from build123d import *

# Parameters (mm, degrees)
SKETCH_1_W          = 51.2
SKETCH_1_H          = 48
EXTRUDE_1_DEPTH     = 120
FILLET_1_R          = 10
SKETCH_3_R          = 6.803864169
EXTRUDE_2_DEPTH     = 10
SKETCH_4_R          = 32
EXTRUDE_3_DEPTH     = 32.5
SKETCH_5_W          = 48
SKETCH_5_H          = 35
CUT_EXTRUDE_1_DEPTH = 178.007598707
SKETCH_6_W          = 6
SKETCH_6_H          = 120
EXTRUDE_6_DEPTH     = 4


with BuildPart() as part:
    # Sketch 1 → Extrude 1 (new body)
    with BuildSketch(Plane(origin=(0, 0, 0), x_dir=(1, 0, 0), z_dir=(0, 1, 0))):
        with Locations((25.6, 24)):
            Rectangle(SKETCH_1_W, SKETCH_1_H)
    extrude(amount=EXTRUDE_1_DEPTH)

    # Fillet 1
    fillet_1_edges = [part.edges().sort_by_distance(p)[0] for p in [
        (51.2, 60, -48),
    ]]
    fillet(fillet_1_edges, radius=FILLET_1_R)

    # Sketch 3 → Extrude 2 (add)
    with BuildSketch(Plane.XZ):
        with Locations(Location((13, -12, 0), (0, 0, 270))):
            Circle(SKETCH_3_R)
    extrude_2 = extrude(amount=EXTRUDE_2_DEPTH)

    # Sketch 4 → Extrude 3 (add)
    with BuildSketch(Plane.XZ.offset(10)):
        with Locations(Location((13, -12, 0), (0, 0, 270))):
            Circle(SKETCH_4_R)
    extrude_3 = extrude(amount=EXTRUDE_3_DEPTH)

    # Mirror 1: Extrude 2, Extrude 3 across plane
    add(extrude_2.mirror(Plane(origin=(0, 60, 0), x_dir=(0, 0, 1), z_dir=(0, -1, 0))))
    add(extrude_3.mirror(Plane(origin=(0, 60, 0), x_dir=(0, 0, 1), z_dir=(0, -1, 0))))

    # Sketch 5 → Cut-Extrude 1 (cut, through all)
    with BuildSketch(Plane.ZY):
        with Locations((-24, 60)):
            Rectangle(SKETCH_5_W, SKETCH_5_H)
    extrude(amount=-CUT_EXTRUDE_1_DEPTH, mode=Mode.SUBTRACT)


with BuildPart() as cut_extrude_1_piece_1:
    # of the separate pieces the step leaves, piece 1, a body of its own (cut_extrude_1_pieces)
    add(part.part.solids().sort_by_distance((13, 130, -44))[0])



with BuildPart() as cut_extrude_1_piece_2:
    # of the separate pieces the step leaves, piece 2, a body of its own (cut_extrude_1_pieces)
    add(part.part.solids().sort_by_distance((51.2, 0, -38))[0])


with BuildPart() as cut_extrude_1_piece_1_1:
    add(cut_extrude_1_piece_1.part)

    add(cut_extrude_1_piece_2.part)  # Extrude 6 merges Cut-Extrude 1 piece 2
    # Sketch 6 → Extrude 6 (add)
    with BuildSketch(Plane.ZY):
        with Locations((-21, 60)):
            Rectangle(SKETCH_6_W, SKETCH_6_H)
    extrude(amount=EXTRUDE_6_DEPTH)


solid = cut_extrude_1_piece_1_1.part
Geometry check sheet. Reference: the model listing, model coordinates, mm. A direction names the side the tool comes from. Coordinates: 2 decimals unless noted, no trailing zeros. Write each loop counter-clockwise with the first axis right and the second up, starting at its lowest first coordinate (ties: lowest second). Pieces come first, ordered by that corner, then holes. Notation, with made-up numbers: (58, 89.25) -> (107, 89.25) arc R19 cw to (107, 108.25) -> close; hole circle Ø4 at (-10.75, -0.5). An arc over 180 degrees is marked (long way). One line per question, with ' | ' between items.
1. Set-up check for faces 1 (the flat face through (0, 98, -36)), 2 (the flat face through (25, 21, 0)), 3 (the flat face through (0, 60, -21)), 4 (the flat face through (-2, 59, -18)), 5 (the cylindrical face through (-15.39, -26.022, -26.766)): record each of +Z, -Z, +X, -X, +Y, -Y from which the full face is reachable in a straight line by a thin tool's end or side.
Answers:
face 1: -Z, -X | face 2: +Z, +X, -X | face 3: +Z, -Z, +X | face 4: +Z, -X | face 5: -Y
2. Cross-section at B-B on z = -12. Record the cut outline in (x, y), and give its area (3 significant figures).
Answers:
outline: (-19, -42.5) -> (45, -42.5) -> (45, -10) -> (19.8, -10) -> (19.8, 0) -> (51.2, 0) -> (51.2, 42.5) -> (0, 42.5) -> (0, 0) -> (6.2, 0) -> (6.2, -10) -> (-19, -10) -> close; (-19, 130) -> (6.2, 130) -> (6.2, 120) -> (0, 120) -> (0, 77.5) -> (51.2, 77.5) -> (51.2, 120) -> (19.8, 120) -> (19.8, 130) -> (45, 130) -> (45, 162.5) -> (-19, 162.5) -> close | area: 8,780 mm²
3. Cross-section at C-C on x = 3.5. Record the cut outline in (y, z).
Answers:
outline: (-42.5, -42.56) -> (-10, -42.56) -> (-10, 18.56) -> (-42.5, 18.56) -> close; (0, -48) -> (42.5, -48) -> (42.5, 0) -> (0, 0) -> close; (77.5, -48) -> (120, -48) -> (120, 0) -> (77.5, 0) -> close; (130, -42.56) -> (162.5, -42.56) -> (162.5, 18.56) -> (130, 18.56) -> close
4. Cross-section at D-D on y = 33.5. Record the cut outline in (x, z), and give its area (3 significant figures).
Answers:
outline: (-4, -24) -> (0, -24) -> (0, -48) -> (41.2, -48) arc R10 ccw to (51.2, -38) -> (51.2, 0) -> (0, 0) -> (0, -18) -> (-4, -18) -> close | area: 2,460 mm²
5. Thickness scan on probe 1 along Y at (x, z) = (15.5, -1); probe 2 along Y at (x, z) = (-13.5, -29.5); probe 3 along Y at (x, z) = (7, -45). Record the ranges inside material, lowest first. Write a range as from..to.
Answers:
probe 1: y = -42.5..-10, 0..42.5, 77.5..120, 130..162.5 | probe 2: y = -42.5..-10, 130..162.5 | probe 3: y = 0..42.5, 77.5..120
6. Draft check along Y on faces 6 (the flat face through (0, 21, -36)), 7 (the flat face through (13, 162.5, -12)), 8 (the cylindrical face through (48.35, 21.55, -44.99)). Enter one of: +Y half, -Y half, draft (parallel to the pull), parting line (faces both ways), or undercut.
Answers:
face 6: undercut | face 7: +Y half | face 8: draft
7. Depth check by flat-ended pin: pin 1 Ø3 at (x, y) = (2.5, 24.5) entering from +Z; pin 2 Ø20 at (y, z) = (12, -7) entering from -X; pin 3 Ø10 at (x, y) = (-3, 110.5) entering from -Z; pin 4 Ø2 at (y, z) = (135.5, -6) entering from -X. Enter the tip coordinate at first touch or a pass-through.
Answers:
pin 1: stops at z = 0 | pin 2: stops at x = 0 | pin 3: stops at z = -48 | pin 4: stops at x = -18.61
8. Cross-section at A-A on x = 13. Record the cut outline in (y, z), and give its area (3 significant figures).
Answers:
outline: (-42.5, -44) -> (-10, -44) -> (-10, -18.8) -> (0, -18.8) -> (0, -48) -> (42.5, -48) -> (42.5, 0) -> (0, 0) -> (0, -5.2) -> (-10, -5.2) -> (-10, 20) -> (-42.5, 20) -> close; (77.5, -48) -> (120, -48) -> (120, -18.8) -> (130, -18.8) -> (130, -44) -> (162.5, -44) -> (162.5, 20) -> (130, 20) -> (130, -5.2) -> (120, -5.2) -> (120, 0) -> (77.5, 0) -> close | area: 8,510 mm²
